Geometry check sheet. Reference: the model listing, model coordinates, mm. A direction names the side the tool comes from. Coordinates: 2 decimals unless noted, no trailing zeros. Write each loop counter-clockwise with the first axis right and the second up, starting at its lowest first coordinate (ties: lowest second). Pieces come first, ordered by that corner, then holes. Notation, with made-up numbers: (63.5, 32.5) -> (122.5, 32.5) arc R15 ccw to (122.5, 54.5) -> close; hole circle Ø3 at (25, 57). An arc over 180 degrees is marked (long way). One line per question, with ' | ' between items.
from build123d import *

# Parameters (mm, degrees)
F3_SIZE  = 10
F4_DEPTH = 25
F5_R     = 7
F6_DEPTH = 25
F7_SIZE  = 2
F8_SIZE  = 1


with BuildPart() as f1:
    # F0 (on Front) → F1 (revolve)
    with BuildSketch(Plane.XZ):
        Polygon((-50, 0), (0, 0), (0, 4), (20, 4), (20, 15), (-50, 15), align=None)
    revolve(axis=Axis((-25, 0, 0), (1, 0, 0)))

    # F3
    f3_edges = [f1.edges().sort_by_distance(p)[0] for p in [
        (-50, 0, -15),
    ]]
    chamfer(f3_edges, length=F3_SIZE)

    # F2 (on Front) → F4 (cut, symmetric)
    with BuildSketch(Plane.XZ):
        Polygon((-60.617507, 4), (-60.617507, 0), (-60.617507, -4), (-60.617507, -15), (-10, -15), (-10, -10), (-55.020042, -10), (-55.020042, -4), (-10, -4), (-10, -2), (-10, 2), (-10, 4), (-55.020042, 4), (-55.020042, 10), (-10, 10), (-10, 15), (-60.617507, 15), align=None)
    extrude(amount=F4_DEPTH, both=True, mode=Mode.SUBTRACT)

    # F5 (on Top) → F6 (cut, symmetric)
    with BuildSketch(Plane.XY):
        with Locations((-30, 0)):
            Circle(F5_R)
    extrude(amount=F6_DEPTH, both=True, mode=Mode.SUBTRACT)

    # F7
    f7_edges = [f1.edges().sort_by_distance(p)[0] for p in [
        (20, 0, -15),
    ]]
    chamfer(f7_edges, length=F7_SIZE)

    # F8
    f8_edges = [f1.edges().sort_by_distance(p)[0] for p in [
        (20, 0, -4),
    ]]
    chamfer(f8_edges, length=F8_SIZE)


solid = f1.part
1. Cross-section at C-C on x = -30. Record the boundary of the cut face in (y, z).
Worked answers:
outline: (-14.46, -4) arc R15 ccw to (-11.18, -10) -> (-7, -10) -> (-7, -4) -> close; (-14.46, 4) -> (-7, 4) -> (-7, 10) -> (-11.18, 10) arc R15 ccw to start; (7, -10) -> (11.18, -10) arc R15 ccw to (14.46, -4) -> (7, -4) -> close; (7, 4) -> (14.46, 4) arc R15 ccw to (11.18, 10) -> (7, 10) -> close
2. Tool access check on faces 4 (the face through (-10, 0, -12)), 5 (the face through (-24, 5, 10)), 6 (the face through (9.633, 3.905, -0.867)), 7 (the face through (20, 0, -6)), 8 (the face through (-10, 0, 0)). Record the directions out of +Z, -Z, +X, -X, +Y, -Y that give a thin tool (end or side, any length) a straight path to the whole face; none if there is none.
Worked answers:
face 4: -Z, -X, +Y, -Y | face 5: +Z, -X, +Y, -Y | face 6: +X | face 7: +Z, -Z, +X, +Y, -Y | face 8: -X, +Y, -Y
3. Mould release check, pull along Y, two halves, no side actions. Record for faces 1 (the face through (-10, 0, 12)), 2 (the face through (-47, 0, -8)), 3 (the face through (-23.323, 2.103, -6.958)): released by +Y, released by -Y, zero draft, split by the parting line, or undercut.
Worked answers:
face 1: zero draft | face 2: split by the parting line | face 3: undercut
4. Cross-section at A-A on x = -38. Record the boundary of the cut face in (y, z), and give its area (3 significant figures).
Worked answers:
outline: (-14.46, -4) arc R15 ccw to (-11.18, -10) -> (11.18, -10) arc R15 ccw to (14.46, -4) -> close; (-14.46, 4) -> (14.46, 4) arc R15 ccw to (11.18, 10) -> (-11.18, 10) arc R15 ccw to start | area: 315 mm²
5. Material ranges on line 1 (Z direction, x = -43.5, y = 1.5); line 2 (Y direction, x = 14.5, z = 0); line 3 (Y direction, x = -30, z = -6.7), recorded low to high. Write a range as from..to.
Worked answers:
line 1: -10..-4, 4..10 | line 2: -15..-4, 4..15 | line 3: -13.42..-7, 7..13.42
6. Cross-section at D-D on z = 0. Record the boundary of the cut face in (x, y).
Worked answers:
outline: (-10, -15) -> (18, -15) -> (20, -13) -> (20, -5) -> (19, -4) -> (0, -4) -> (0, 4) -> (19, 4) -> (20, 5) -> (20, 13) -> (18, 15) -> (-10, 15) -> close
7. Go/stop test with flat-tipped pins: P1, Ø6.5, axis at y = 0, z = 0, coming from the -X side; P2, Ø14.5, axis at x = -34, y = 5.5, coming from the +Z side; P3, Ø5, axis at x = -17.5, z = -2, coming from the +Y side. Record where each tip stops, or that it passes through.
Worked answers:
P1: x = -10 | P2: z = 10 | P3: y = 14.46
8. Cross-section at B-B on y = 0. Give the number of separate pieces and of enclosed holes in the cut face, and give its area (3 significant figures).
Worked answers:
separate pieces: 3 | enclosed holes: 0 | area: 1,020 mm²
